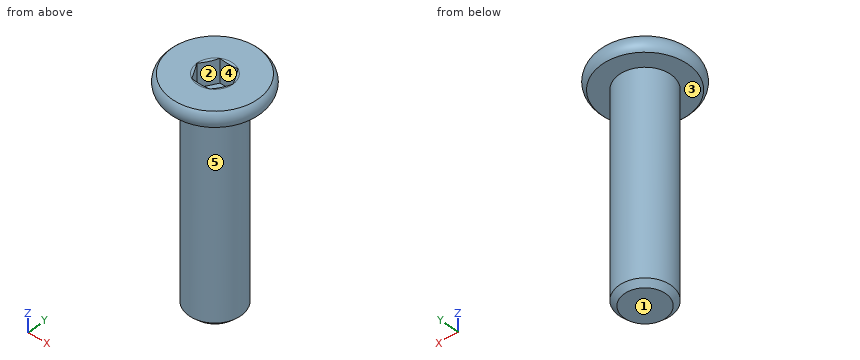
Autodesk Inventor part; units mm, degrees
ref_plane "YZ Plane" through (0, 0, 0) normal (1, 0, 0) x (0, 1, 0)
ref_plane "XZ Plane" through (0, 0, 0) normal (0, 1, 0) x (-1, 0, 0)
ref_plane "XY Plane" through (0, 0, 0) normal (0, 0, 1) x (1, 0, 0)
sketch "Sketch1" plane through (0, 0, 0) normal (1, 0, 0) x (0, 1, 0)
  line L0 (2.5, 2.81) -> (2.5, 11.31)
  spline S0 degree 2 poles (-3.9658, 2.81) (-4.0258, 2.8689) (-4.0876, 2.9295) knots 0 0 0 0.017848 0.017848 0.017848 weights 1 1.00044 1.00066
  line L1 (-2.5, 11.31) -> (-2.5, 2.81)
  line L2 (1.7321, 14.76) -> (1.7821, 14.81)
  line L3 (-1.7821, 14.81) -> (4.1614, 14.81)
  arc A0 (4.1614, 13.31) -> (4.1614, 14.81) centre (3.5, 14.06) ccw
  line L4 (4.1614, 13.31) -> (2.5, 13.31)
  line L5 (2.5, 13.31) -> (2.5, -6.19)
  line L6 (-2.5, -6.19) -> (-2.5, 13.31)
  line L7 (-2.5, 13.31) -> (-4.1614, 13.31)
  arc A1 (-4.1614, 14.81) -> (-4.1614, 13.31) centre (-3.5, 14.06) ccw
  line L8 (-4.1614, 14.81) -> (-1.7821, 14.81)
  line L9 (-1.7821, 14.81) -> (-1.7321, 14.76)
  line L10 (0, -6.69) -> (0, 14.81)
  line L11 (-2, -6.69) -> (2, -6.69)
  line L12 (2.5, -6.19) -> (2, -6.69)
  line L13 (-2.5, -6.19) -> (-2, -6.69)
  point P0 (0, 0)
  point P1 (2.5, -6.69)
  point P2 (-2.5, -6.69)
  dimension "d10" = 0.5
  dimension "d11" = 0.5
  dimension "d12" = 0.5
  dimension "d13" = 0.5
revolve "Revolution1" add sketch "Sketch1" angle 360 about axis through (0, 0, -6.69) along (0, 0, 1) contours L5 L12 L11 L10 L3 A0 L4 L0
sketch "Sketch2" plane through (0, 0, 14.81) normal (0, 0, 1) x (1, 0, 0)
  line L0 (1.732, 0) -> (0.866, -1.5)
  line L1 (0.866, -1.5) -> (-0.866, -1.5)
  line L2 (-0.866, -1.5) -> (-1.732, 0)
  line L3 (-1.732, 0) -> (-0.866, 1.5)
  line L4 (-0.866, 1.5) -> (0.866, 1.5)
  line L5 (0.866, 1.5) -> (1.732, 0)
  point P0 (0, 0)
  point P1 (0, 0)
  dimension "d1" = 3.464
extrude "Extrusion1" cut sketch "Sketch2" against normal blind 2.3
sketch "Sketch3" plane through (0, 0, 0) normal (0, 1, 0) x (-1, 0, 0)
  line L0 (0.866, 14.81) -> (-0.866, 14.81)
  line L1 (0.866, 14.81) -> (0.866, 12.51)
  line L2 (0.866, 12.51) -> (-0.866, 12.51)
  line L3 (-0.866, 14.81) -> (-0.866, 12.51)
  line L4 (1.732, 14.81) -> (1.732, 12.51)
  circle A0 centre (0, 19.6597) radius 5.1497
  line L5 (0, 14.81) -> (0, 14.51)
  line L6 (0, 14.81) -> (0, 24.8094)
  point P0 (0, 0)
  dimension "d5" = 0.3
revolve "Revolution2" cut sketch "Sketch3" angle 360 about axis through (0, 0, 14.81) along (0, 0, 1) contours L5 A0 L3 L0 | L0 L3 A0 L6
thread "Thread1"
properties part number "Low Profile Screw M5 [20mm]" material "Steel"
The model under review builds one solid part; all positions refer to its coordinate system, in mm. Face numbers are marked on the shaded views. A direction names the side the tool comes from. Round coordinates to 2 decimals unless told otherwise and drop trailing zeros. Loops run counter-clockwise (first coordinate to the right, second up) from the corner with the lowest first, then second, coordinate; pieces in that order, holes last. Notation, with made-up numbers: M 50,-22 L 101,-22 A26 cw 101,2 Z; hole C 86,86.5 d10. An arc over 180 degrees is marked long. Answer as a JSON object with one key per item and string values.
Item 1: Clearance check with flat-ended pins moving along their axes: P1, Ø1.4, axis at x = -0.5, z = 13.5, coming from the -Y side; P2, Ø0.5, axis at x = 0, z = 13.5, coming from the +Y side; P3, Ø1.5, axis at x = 0, y = -0.5, coming from the +Z side; P4, Ø3, axis at x = 3.5, z = 3, coming from the -Y side. State where each tip first meets the part, or that it passes through.
Check sheet entries:
{"P1": "y = -4.5", "P2": "y = 4.45", "P3": "z = 12.51", "P4": "y = -1.5"}
Item 2: The part is to be moulded in two halves that separate along X. For the marked faces 3, 4 and 5, say which applies: +X half, -X half, draft (parallel to the pull), parting line (faces both ways), or undercut.
Check sheet entries:
{"face 3": "draft", "face 4": "undercut", "face 5": "parting line"}
Item 3: For line 1 along Z through (x, y) = (-0.5, -3.5); line 2 along X through (y, z) = (2, 11.5); line 3 along Y through (x, z) = (-1.5, 1), list the stretches that pass through material, from the lowest coordinate up.
Check sheet entries:
{"line 1": "13.31 to 14.81", "line 2": "-1.5 to 1.5", "line 3": "-2 to 2"}
Item 4: We need section A-A, the plane z = 8. State the section outline as (x, y) points.
Check sheet entries:
{"outline": "C 0,0 d5"}
Item 5: Tool access review of the marked faces 1 and 2: name each direction out of +Z, -Z, +X, -X, +Y, -Y from which nothing blocks a thin tool from reaching the whole face with its end or side.
Check sheet entries:
{"face 1": "-Z, +X, -X, +Y, -Y", "face 2": "+Z"}
